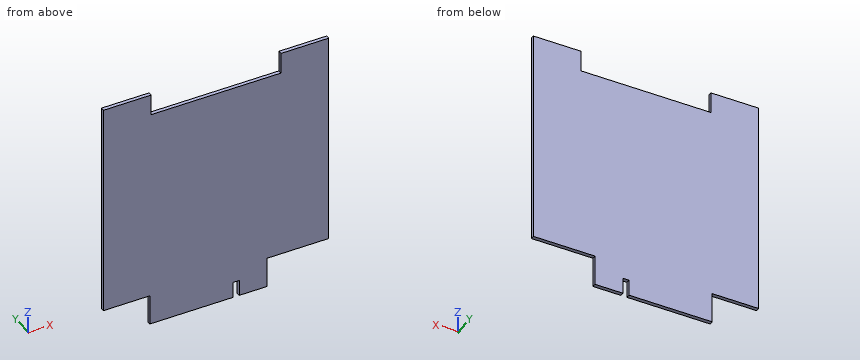
from build123d import *

# Parameters (mm, degrees)
SKETCH1_W           = 49.880837057
SKETCH1_H           = 12.780388143
SKETCH1_W_2         = 95.885
SKETCH1_H_2         = 90.805
BOSS_EXTRUDE1_DEPTH = 1.6
SKETCH2_W           = 55.245
SKETCH2_H           = 8.89
SKETCH2_W_2         = 2.610734202
SKETCH2_H_2         = 6.76
CUT_EXTRUDE1_DEPTH  = 1.6


with BuildPart() as part:
    # Sketch1 → Boss-Extrude1 (new body)
    with BuildSketch(Plane(origin=(0, 0, 0), x_dir=(1, 0, 0), z_dir=(0, 1, 0))):
        with Locations((-3.227112148, 51.792694072)):
            Rectangle(SKETCH1_W, SKETCH1_H)
        Rectangle(SKETCH1_W_2, SKETCH1_H_2)
    extrude(amount=BOSS_EXTRUDE1_DEPTH)

    # Sketch2 → Cut-Extrude1 (cut)
    with BuildSketch(Plane(origin=(0, 1.6, 0), x_dir=(1, 0, 0), z_dir=(0, 1, 0))):
        with Locations((0, -40.9575)):
            Rectangle(SKETCH2_W, SKETCH2_H)
        with Locations((8.587941455, 54.802888143)):
            Rectangle(SKETCH2_W_2, SKETCH2_H_2)
    extrude(amount=-CUT_EXTRUDE1_DEPTH, mode=Mode.SUBTRACT)


solid = part.part
Source: CAD feature listing. Evaluate the final solid. Frame: model axes, mm. Round coordinates to 2 decimals unless told otherwise and drop trailing zeros. Loops run counter-clockwise (first coordinate to the right, second up) from the corner with the lowest first, then second, coordinate; pieces in that order, holes last. Notation, with made-up numbers: (17, 89.25) - (76, 89.25) arc R25 ccw to (76, 101.25) - close; hole circle Ø5 at (28.25, 31). An arc over 180 degrees is marked (long way). Write item = value, one per line. Start each with the question number.
Item 1: First-contact query: pin 1 Ø1 at (x, z) = (37.5, -46.5) entering from +Y; pin 2 Ø0.8 at (y, z) = (0.5, -50) entering from -X; pin 3 Ø0.5 at (x, y) = (-39, 1) entering from -Z; pin 4 Ø0.5 at (y, z) = (1, -53) entering from +X. Flat tips, straight axial feed; report the tip coordinate or a pass-through.
Item 2: Section query B-B on x = -6. Output: boundary loops of the cut face in (y, z), plus the area to 3 significant figures.
Item 3: Material intervals for line 1 (Z direction, x = -42.5, y = 1.55); line 2 (Z direction, x = 14, y = 0.1), sorted ascending.
Item 4: Section query A-A on y = 0.45. Output: boundary loops of the cut face in (x, z).
Results list:
q1.pin_1 = through
q1.pin_2 = -28.17
q1.pin_3 = -45.4
q1.pin_4 = 21.71
q2.outline = (0, -58.18) - (1.6, -58.18) - (1.6, 36.51) - (0, 36.51) - close
q2.area = 152 mm²
q3.line_1 = -45.4 to 45.4
q3.line_2 = -58.18 to 36.51
q4.outline = (-47.94, -45.4) - (-28.17, -45.4) - (-28.17, -58.18) - (7.28, -58.18) - (7.28, -51.42) - (9.89, -51.42) - (9.89, -58.18) - (21.71, -58.18) - (21.71, -45.4) - (47.94, -45.4) - (47.94, 45.4) - (27.62, 45.4) - (27.62, 36.51) - (-27.62, 36.51) - (-27.62, 45.4) - (-47.94, 45.4) - close
